from build123d import *

# Parameters (mm, degrees)
SKETCH1_W           = 5
SKETCH1_H           = 50
BOSS_EXTRUDE1_DEPTH = 200
CUT_EXTRUDE2_DEPTH  = 5
CHAMFER1_SIZE       = 5
SKETCH2_R           = 2
CUT_EXTRUDE1_DEPTH  = 5
SKETCH4_R           = 2
CUT_EXTRUDE3_DEPTH  = 5


with BuildPart() as part:
    # Sketch1 → Boss-Extrude1 (new body)
    with BuildSketch(Plane(origin=(0, 0, 0), x_dir=(0, 0, -1), z_dir=(1, 0, 0))):
        with Locations((-2.5, 25)):
            Rectangle(SKETCH1_W, SKETCH1_H)
    extrude(amount=BOSS_EXTRUDE1_DEPTH)

    # Sketch3 → Cut-Extrude2 (cut)
    with BuildSketch(Plane.XY.offset(5)):
        Polygon((0, 50), (200, 50), (200, 32.502267295), align=None)
    extrude(amount=-CUT_EXTRUDE2_DEPTH, mode=Mode.SUBTRACT)

    # Chamfer1
    chamfer1_edges = [part.edges().sort_by_distance(p)[0] for p in [
        (100, 41.251133647, 0),
    ]]
    chamfer(chamfer1_edges, length=CHAMFER1_SIZE - 0.0001)  # a hair under: the kernel refuses the full size

    # Sketch2 → Cut-Extrude1 (cut)
    with BuildSketch(Plane(origin=(0, 0, 0), x_dir=(-1, 0, 0), z_dir=(0, 0, -1))):
        with Locations((-192, 8)):
            Circle(SKETCH2_R)
        with Locations((-180, 8)):
            Circle(SKETCH2_R)
    cut_extrude1 = extrude(amount=-CUT_EXTRUDE1_DEPTH, mode=Mode.SUBTRACT)

    # Mirror2: Cut-Extrude1 across plane
    add(cut_extrude1.mirror(Plane(origin=(100, 0, 0), x_dir=(0, 0, 1), z_dir=(1, 0, 0))), mode=Mode.SUBTRACT)

    # Sketch4 → Cut-Extrude3 (cut)
    with BuildSketch(Plane(origin=(0, 0, 0), x_dir=(-1, 0, 0), z_dir=(0, 0, -1))):
        with Locations(Location((-80, 8, 0), (0, 0, 90))):
            Circle(SKETCH4_R)
        with Locations(Location((-96, 8, 0), (0, 0, 90))):
            Circle(SKETCH4_R)
    extrude(amount=-CUT_EXTRUDE3_DEPTH, mode=Mode.SUBTRACT)


solid = part.part
The listing builds one solid part. Answer for the finished solid, in the listing's coordinates (mm). Round coordinates to 2 decimals unless told otherwise and drop trailing zeros. Write each loop counter-clockwise with the first axis right and the second up, starting at its lowest first coordinate (ties: lowest second). Pieces come first, ordered by that corner, then holes. Notation, with made-up numbers: M -27.5,56.5 L 9.5,56.5 A8 cw 9.5,63.5 Z; hole C 69,53.5 d7. An arc over 180 degrees is marked long. Write each question's results on one line, items separated by ' | '. Start each with the question number.
Item 1: For a pull along Y with two mould halves and no side action, classify faces 1 (the face through (99, 0, 3)), 2 (the face through (6.526, 9.352, 2.465)), 3 (the face through (99, 19, 5)) as pulls with the +Y half, pulls with the -Y half, needs draft (parallel to the pull), parting line crosses it, or undercut.
Item 2: Straight lines are drawn through the part: L1, parallel to Y at x = 180, z = 1.5; L2, parallel to Y at x = 46.5, z = 4.05; L3, parallel to Y at x = 169, z = 1.4. For each, find the intervals that lie inside material, in ascending order. Write a range as [from, to].
Item 3: Flat-ended cylindrical pins translate along their axes: pin 1 Ø3 at (x, z) = (107, 2) entering from +Y; pin 2 Ø5 at (x, y) = (192, 8) entering from +Z. Find the tip coordinate at first contact, or state that the pin passes through.
Item 4: A cutting plane is placed at B-B on z = 2.5. Write down the section's boundary in (x, y), and give its area (3 significant figures).
Check sheet entries:
1) face 1: pulls with the -Y half | face 2: undercut | face 3: needs draft
2) L1: [0, 6], [10, 30.74] | L2: [0, 44.98] | L3: [0, 31.6]
3) pin 1: y = 39.14 | pin 2: z = 5
4) outline: M 0,0 L 200,0 L 200,29.99 L 0,47.49 Z; hole C 8,8 d4; hole C 20,8 d4; hole C 80,8 d4; hole C 96,8 d4; hole C 180,8 d4; hole C 192,8 d4 | area: 7,670 mm²
